Here's how the part is built. I have some questions about the finished solid (model axes, mm). Face numbers are marked on the shaded views. A direction names the side the tool comes from. Coordinates: 2 decimals unless noted, no trailing zeros. Loops run counter-clockwise (first coordinate to the right, second up) from the corner with the lowest first, then second, coordinate; pieces in that order, holes last. Notation, with made-up numbers: (27.25, 45.25) - (43.25, 45.25) arc R36 ccw to (43.25, 79.25) - close; hole circle Ø11 at (-21.5, 67). An arc over 180 degrees is marked (long way). Use a Markdown table: item, result.
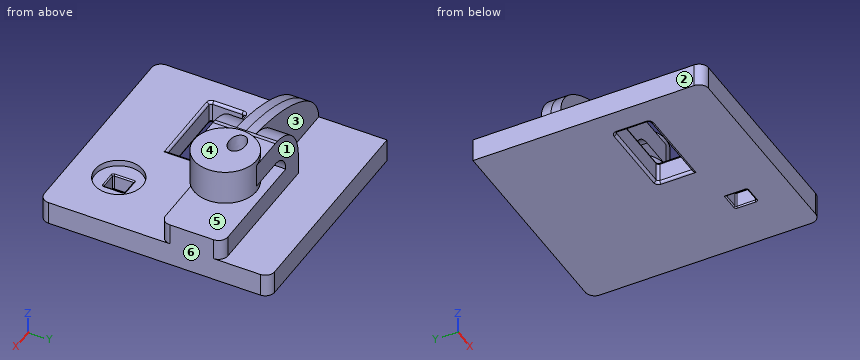
```python
from build123d import *

# Parameters (mm, degrees)
F1_DEPTH  = 63.5
F0_W      = 25.4
F0_H      = 19.05
F2_DEPTH  = 25.4
F3_DEPTH  = 7.9375
F5_DEPTH  = 95.25
F6_DEPTH  = 60.706
F7_W      = 64.0991125256
F7_H      = 28.2470658422
F8_DEPTH  = 25.4
F9_R      = 19.5079134093
F10_DEPTH = 5.08
F11_W     = 14.4394114614
F11_H     = 16.9663056731
F12_DEPTH = 25.4
F14_DEPTH = 28.575
F15_R     = 7.62
F16_R     = 2.032
F17_R     = 1.016


with BuildPart() as f1:
    # F0 (on Front) → F1 (new body, symmetric)
    with BuildSketch(Plane.XZ):
        Polygon((22.225, 9.525), (-41.275, 9.525), (-41.275, -9.525), (41.275, -9.525), (41.275, 9.525), align=None)
    extrude(amount=F1_DEPTH, both=True)

    # F0 (on Front) → F2 (join, symmetric)
    with BuildSketch(Plane.XZ):
        with BuildLine():
            Line((22.225, 27.0002), (22.225, 9.525))
            Line((22.225, 9.525), (41.275, 9.525))
            Line((41.275, 9.525), (41.275, 27.0002))
            ThreePointArc((41.275, 27.0002), (45.9246798487, 38.2255201513), (57.15, 42.8752))
            Line((57.15, 42.8752), (60.325, 42.8752))
            Line((60.325, 42.8752), (60.325, 61.9252))
            Line((60.325, 61.9252), (57.15, 61.9252))
            add(Edge.make_bspline(
                [(53.8854342407, 61.7722898912), (54.9842067368, 61.8365871986), (56.0728453275, 61.8876096574), (57.15, 61.9252)],
                knots=[108.5245810491, 108.5245810491, 108.5245810491, 108.5245810491, 111.5045361635, 111.5045361635, 111.5045361635, 111.5045361635], degree=3))
            ThreePointArc((53.8854342407, 61.7722898912), (31.3258777096, 50.5133948686), (22.225, 27.0002))
        make_face()
        with Locations((73.025, 52.4002)):
            Rectangle(F0_W, F0_H)
    extrude(amount=F2_DEPTH, both=True)

    # F0 (on Front) → F3 (join, symmetric)
    with BuildSketch(Plane.XZ):
        with BuildLine():
            add(Edge.make_bspline(
                [(-41.275, 9.525), (-39.5856284224, 39.4828766469), (13.870125209, 59.4306981306), (53.8854342407, 61.7722898912)],
                knots=[0, 0, 0, 0, 108.5245810491, 108.5245810491, 108.5245810491, 108.5245810491], degree=3))
            Line((-41.275, 9.525), (22.225, 9.525))
            Line((22.225, 9.525), (22.225, 27.0002))
            ThreePointArc((22.225, 27.0002), (31.3258777096, 50.5133948686), (53.8854342407, 61.7722898912))
        make_face()
    extrude(amount=F3_DEPTH, both=True)

    # F0 (on Front) → F4 (revolve)
    with BuildSketch(Plane.XZ):
        Polygon((85.725, 66.675), (85.725, 61.9252), (85.725, 42.8752), (85.725, 38.1), (111.125, 38.1), (111.125, 66.675), align=None)
    revolve(axis=Axis((85.725, 0, 52.3875), (0, 0, 1)))

    # F5 (add): a face of the model
    f5_faces = [f1.faces().sort_by_distance(p)[0] for p in [
        (41.275, 0, 4.9023288334),
    ]]
    extrude(f5_faces, amount=F5_DEPTH)

    # F6 (add): a face of the model
    f6_faces = [f1.faces().sort_by_distance(p)[0] for p in [
        (47.625, -63.5, 0),
    ]]
    extrude(f6_faces, amount=F6_DEPTH)

    # F7 (on face) → F8 (cut)
    with BuildSketch(Plane.XY.offset(9.525)):
        with Locations((12.3161775991, -54.8000894487)):
            Rectangle(F7_W, F7_H)
    extrude(amount=-F8_DEPTH, mode=Mode.SUBTRACT)

    # F9 (on face) → F10 (cut)
    with BuildSketch(Plane.XY.offset(9.525)):
        with Locations((87.4239131329, -85.8199995224)):
            Circle(F9_R)
    extrude(amount=-F10_DEPTH, mode=Mode.SUBTRACT)

    # F11 (on face) → F12 (cut)
    with BuildSketch(Plane.XY.offset(9.525)):
        with Locations((88.0553610623, -85.5649597943)):
            Rectangle(F11_W, F11_H)
    extrude(amount=-F12_DEPTH, mode=Mode.SUBTRACT)

    # F13 (on face) → F14 (cut, through all)
    with BuildSketch(Plane.XY.offset(66.675)):
        with BuildLine():
            add(Edge.make_bspline(
                [(84.4615474343, 3.9708414115), (84.4615474343, 15.3508284031), (69.8416419327, 9.6608349073), (55.2217364311, 3.9708414115), (69.8416419327, -1.7191520843), (84.4615474343, -7.4091455801), (84.4615474343, 3.9708414115)],
                knots=[0, 0, 0, 2.0943951024, 2.0943951024, 4.1887902048, 4.1887902048, 6.2831853072, 6.2831853072, 6.2831853072], degree=2, weights=[1, 0.5, 1, 0.5, 1, 0.5, 1]))
        make_face()
    extrude(amount=-F14_DEPTH, mode=Mode.SUBTRACT)

    # F15
    f15_edges = [f1.edges().sort_by_distance(p)[0] for p in [
        (-41.275, -124.206, 0),
        (136.525, -124.206, 0),
        (136.525, -25.4, 18.2626),
        (136.525, 25.4, 18.2626),
        (136.525, 63.5, 0),
    ]]
    fillet(f15_edges, radius=F15_R)

    # F16
    f16_edges = [f1.edges().sort_by_distance(p)[0] for p in [
        (-19.733379, -54.800089, 9.525),
        (-19.733379, -68.923622, 0),
        (-19.733379, -54.800089, -9.525),
        (-19.733379, -40.676557, 0),
        (12.316178, -40.676557, 9.525),
        (12.316178, -40.676557, -9.525),
        (44.365734, -40.676557, 0),
        (12.316178, -68.923622, -9.525),
        (44.365734, -54.800089, -9.525),
        (12.316178, -68.923622, 9.525),
        (44.365734, -54.800089, 9.525),
    ]]
    fillet(f16_edges, radius=F16_R)

    # F17
    f17_edges = [f1.edges().sort_by_distance(p)[0] for p in [
        (88.055361, -77.081807, 4.445),
        (95.275067, -85.56496, 4.445),
        (95.275067, -77.081807, -2.54),
        (95.275067, -85.56496, -9.525),
        (95.275067, -94.048113, -2.54),
        (80.835655, -85.56496, 4.445),
        (88.055361, -94.048113, 4.445),
        (88.055361, -94.048113, -9.525),
        (80.835655, -94.048113, -2.54),
        (80.835655, -85.56496, -9.525),
        (88.055361, -77.081807, -9.525),
    ]]
    fillet(f17_edges, radius=F17_R)


solid = f1.part
```
Q1. If we mould it in two halves opening along Z, with no side actions, what happens to the marked faces 4, 5 and 6? For each: pulls with the +Z half, pulls with the -Z half, needs draft (parallel to the pull), parting line crosses it, or undercut.
Check values:
| item | result |
|---|---|
| face 4 | pulls with the +Z half |
| face 5 | undercut |
| face 6 | needs draft |
Q2. Which directions (+Z, -Z, +X, -X, +Y, -Y) give clear straight access to the entire face, cutting with the end or side of a thin tool? Please do the marked faces 1, 2 and 3.
Check values:
| item | result |
|---|---|
| face 1 | +Z, +X, -X, +Y |
| face 2 | +Z, -Z, -X, +Y, -Y |
| face 3 | +Z, -X, +Y |
Q3. I want a section at A-A, the plane y = -85.82. Write out the boundary of the cut face in (x, z) (3 decimals), then the cut area to 3 significant figures.
Check values:
| item | result |
|---|---|
| outline | (-41.275, -9.525) - (79.82, -9.525) arc R1.016 ccw to (80.836, -8.509) - (80.836, 3.429) arc R1.016 ccw to (79.82, 4.445) - (67.916, 4.445) - (67.916, 9.525) - (-41.275, 9.525) - close; (95.275, -8.509) arc R1.016 ccw to (96.291, -9.525) - (136.525, -9.525) - (136.525, 9.525) - (106.932, 9.525) - (106.932, 4.445) - (96.291, 4.445) arc R1.016 ccw to (95.275, 3.429) - close |
| area | 2,990 mm^2 |
Q4. Please list where these lines run through material, in increasing order: L1, parallel to Y at x = -8, z = 25; L2, parallel to Z at x = 89, y = -1 (3 decimals); L3, parallel to Z at x = 59.5, y = 14.5 (3 decimals). Write a range as from..to.
Check values:
| item | result |
|---|---|
| L1 | -7.94..7.94 |
| L2 | -9.525..27, 38.1..66.675 |
| L3 | -9.525..27, 42.875..61.925 |
Q5. Will these pins go through, and if not, where does the flat tip stop? P1, Ø5, axis at y = 12.5, z = 17.5, coming from the -X side (3 decimals); P2, Ø10, axis at x = 21.5, y = -71, coming from the +Z side (3 decimals); P3, Ø12, axis at x = 90, y = -74.5, coming from the +Z side (3 decimals).
Check values:
| item | result |
|---|---|
| P1 | x = 22.225 |
| P2 | z = 9.525 |
| P3 | z = 4.445 |
Q6. I want a section at B-B, the plane z = 1. Write out the boundary of the cut face in (x, y) (3 decimals).
Check values:
| item | result |
|---|---|
| outline | (-41.275, -116.586) arc R7.62 ccw to (-33.655, -124.206) - (128.905, -124.206) arc R7.62 ccw to (136.525, -116.586) - (136.525, 55.88) arc R7.62 ccw to (128.905, 63.5) - (-41.275, 63.5) - close; hole (-19.733, -66.892) arc R2.032 ccw to (-17.701, -68.924) - (44.366, -68.924) - (44.366, -42.709) arc R2.032 ccw to (42.334, -40.677) - (-17.701, -40.677) arc R2.032 ccw to (-19.733, -42.709) - close; hole (80.836, -93.032) arc R1.016 ccw to (81.852, -94.048) - (94.259, -94.048) arc R1.016 ccw to (95.275, -93.032) - (95.275, -78.098) arc R1.016 ccw to (94.259, -77.082) - (80.836, -77.082) - close |
Q7. I want a section at C-C, the plane y = 37. Write out the boundary of the cut face in (x, z) (3 decimals), then the cut area to 3 significant figures.
Check values:
| item | result |
|---|---|
| outline | (-41.275, -9.525) - (136.525, -9.525) - (136.525, 9.525) - (-41.275, 9.525) - close |
| area | 3,390 mm^2 |
